Here's the drawing with two shaded views (mm, measured from the low corner). I have some questions. A direction names the side the tool comes from. Coordinates: 2 decimals unless noted, no trailing zeros. Write each loop counter-clockwise with the first axis right and the second up, starting at its lowest first coordinate (ties: lowest second). Pieces come first, ordered by that corner, then holes.
Item 1: I want a section at D-D on z = 34. Please give me the cut outline in (x, y).
Item 2: I want a section at C-C on x = 25. Please give me the cut outline in (y, z).
Item 3: Which directions (+Z, -Z, +X, -X, +Y, -Y) give clear straight access to the entire face, cutting with the end or side of a thin tool? Please do the marked faces 5, 6, 7, 8 and 9.
Item 4: I want a section at A-A on y = 11.5. Please give me the cut outline in (x, z).
Item 5: If I drill on probe 1 along X at (y, z) = (2, 37.5); probe 2 along Z at (x, y) = (77.5, 1.7); probe 3 along X at (y, z) = (13, 17.5), over which ranges is the centre line in solid material (lowest first)?
Item 6: For P1, Ø5.5, axis at x = 78, z = 33.5, coming from the +Y side; P2, Ø10, axis at y = 11, z = 15.5, coming from the -X side; P3, Ø3.5, axis at x = 2.5, y = 24, coming from the +Z side; P4, Ø3.5, axis at x = 77, y = 24, coming from the -Z side, each with a flat end and sliding along its axis, tell me the tip position at first contact or that it passes through.
Item 7: I want a section at B-B on z = 11.5. Please give me the cut outline in (x, y).
Item 8: Thinking about a two-plate mould opening in X: for the marked faces 1, 2, 3 and 4, which applies, +X half, -X half, draft (parallel to the pull), parting line (faces both ways), or undercut?
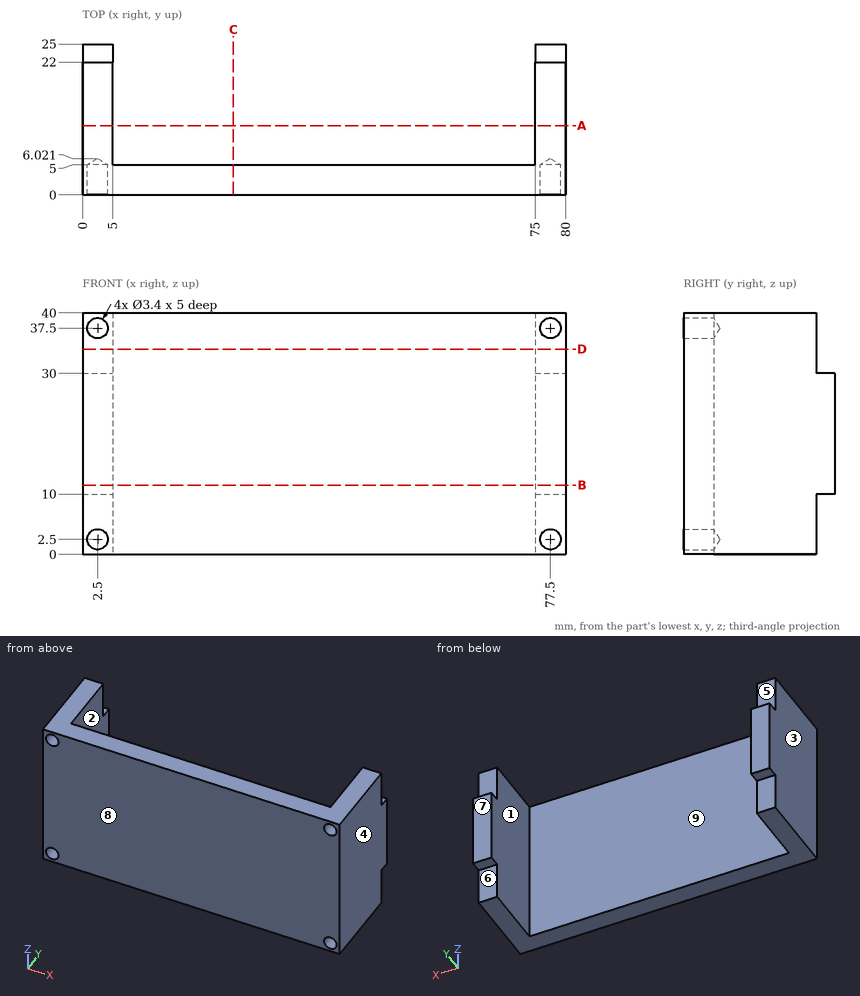
Response values:
1. outline: (0, 0) - (80, 0) - (80, 22) - (75, 22) - (75, 5) - (5, 5) - (5, 22) - (0, 22) - close
2. outline: (0, 0) - (5, 0) - (5, 40) - (0, 40) - close
3. face 5: +Z, +X, -X, +Y
3. face 6: -Z, +X, -X, +Y
3. face 7: +Z, -Z, +X, -X, +Y
3. face 8: +Z, -Z, +X, -X, -Y
3. face 9: +Z, -Z, +Y
4. outline: (0, 0) - (5, 0) - (5, 40) - (0, 40) - close; (75, 0) - (80, 0) - (80, 40) - (75, 40) - close
5. probe 1: x = 0 to 0.8, 4.2 to 75.8, 79.2 to 80
5. probe 2: z = 0 to 0.8, 4.2 to 35.8, 39.2 to 40
5. probe 3: x = 0 to 5, 75 to 80
6. P1: stops at y = 22
6. P2: stops at x = 0
6. P3: stops at z = 30
6. P4: stops at z = 10
7. outline: (0, 0) - (80, 0) - (80, 25) - (75, 25) - (75, 5) - (5, 5) - (5, 25) - (0, 25) - close
8. face 1: undercut
8. face 2: undercut
8. face 3: -X half
8. face 4: +X half
